Design review of the part built by this model. Coordinates are the model's own, in mm. A direction names the side the tool comes from. Coordinates: 2 decimals unless noted, no trailing zeros. Loops run counter-clockwise (first coordinate to the right, second up) from the corner with the lowest first, then second, coordinate; pieces in that order, holes last.
Q1. Add section C-C on x = 31.5. Give the boundary of the cut face in (y, z).
Q2. Draft analysis for pull direction X (two halves, no side actions). For faces 3 (the face through (2.85, 3.19, -81.99)), 4 (the face through (42.3, 0.4, -5)), 5 (the face through (7.008, 3.901, -40.115)), state which applies: released by +X, released by -X, zero draft, split by the parting line, or undercut.
Q3. For P1, Ø1.5, axis at x = 75, y = 4.5, coming from the +Z side; P2, Ø2, axis at x = 76.5, y = 2, coming from the +Z side, all flat-tipped, find the tip position at first contact; note any pin that passes through.
Q4. Add section D-D on y = 3.15. Give the boundary of the cut face in (x, z).
Q5. Add section B-B on z = -16.5. Give the boundary of the cut face in (x, y), and give its area (3 significant figures).
Q6. Wall thickness on probe 1 along X at (y, z) = (4.5, -50); probe 2 along Y at (x, z) = (4, -42.5); probe 3 along X at (y, z) = (4.5, -11.5): over which ranges is each line inside the solid? List them lowest first.
Q7. Machinability: for faces 1 (the face through (85, 3, -47)), 2 (the face through (22.92, 3.19, -23.91)), which of the approach directions +Z, -Z, +X, -X, +Y, -Y give a long, thin tool a straight path to every point of the face, cutting with its end or side? Answer none if there is none.
Q8. Add section A-A on x = 42.5. Give the boundary of the cut face in (y, z).
```python
from build123d import *

# Parameters (mm, degrees)
SKETCH1_W           = 85
SKETCH1_H           = 85
BOSS_EXTRUDE1_DEPTH = 6.3
CUT_EXTRUDE1_DEPTH  = 10
SKETCH3_R           = 2.5
CUT_EXTRUDE2_DEPTH  = 86
SKETCH4_R           = 2.5
CUT_EXTRUDE3_DEPTH  = 86
FILLET1_R           = 20
FILLET2_R           = 10


with BuildPart() as part:
    # Sketch1 → Boss-Extrude1 (new body)
    with BuildSketch(Plane(origin=(0, 0, 0), x_dir=(1, 0, 0), z_dir=(0, 1, 0))):
        with Locations((42.5, 42.5)):
            Rectangle(SKETCH1_W, SKETCH1_H)
    extrude(amount=BOSS_EXTRUDE1_DEPTH)

    # Sketch2 → Cut-Extrude1 (cut)
    with BuildSketch(Plane(origin=(0, 6.3, 0), x_dir=(1, 0, 0), z_dir=(0, 1, 0))):
        with BuildLine():
            Line((16.519237886, 35), (29.509618943, 12.5))
            ThreePointArc((29.509618943, 12.5), (42.5, 5), (55.490381057, 12.5))
            Line((55.490381057, 12.5), (68.480762114, 35))
            ThreePointArc((68.480762114, 35), (42.5, 80), (16.519237886, 35))
        make_face()
    extrude(amount=-CUT_EXTRUDE1_DEPTH, mode=Mode.SUBTRACT)

    # Sketch3 → Cut-Extrude2 (cut, through all)
    with BuildSketch(Plane.XY):
        with Locations((42.5, 3.15)):
            Circle(SKETCH3_R)
    extrude(amount=-CUT_EXTRUDE2_DEPTH, mode=Mode.SUBTRACT)

    # Sketch4 → Cut-Extrude3 (cut, through all)
    with BuildSketch(Plane.ZY):
        with Locations((-42.5, 3.15)):
            Circle(SKETCH4_R)
    extrude(amount=-CUT_EXTRUDE3_DEPTH, mode=Mode.SUBTRACT)

    # Fillet1
    fillet1_edges = [part.edges().sort_by_distance(p)[0] for p in [
        (85, 3.15, 0),
        (0, 3.15, 0),
    ]]
    fillet(fillet1_edges, radius=FILLET1_R)

    # Fillet2
    fillet2_edges = [part.edges().sort_by_distance(p)[0] for p in [
        (0, 3.15, -85),
        (85, 3.15, -85),
    ]]
    fillet(fillet2_edges, radius=FILLET2_R)


solid = part.part
```
Entries:
1. outline: (0, -85) - (6.3, -85) - (6.3, -77.91) - (0, -77.91) - close; (0, -9.8) - (6.3, -9.8) - (6.3, 0) - (0, 0) - close
2. face 3: released by -X
2. face 4: undercut
2. face 5: zero draft
3. P1: stops at z = -2.27
3. P2: stops at z = -2.98
4. outline: (0, -75) arc R10 ccw to (10, -85) - (40, -85) - (40, -79.9) arc R30 cw to (12.92, -45) - (0, -45) - close; (0, -40) - (14.22, -40) arc R30 cw to (16.52, -35) - (29.51, -12.5) arc R15 cw to (40, -5.21) - (40, 0) - (20, 0) arc R20 ccw to (0, -20) - close; (45, -85) - (75, -85) arc R10 ccw to (85, -75) - (85, -45) - (72.08, -45) arc R30 cw to (45, -79.9) - close; (45, -5.21) arc R15 cw to (55.49, -12.5) - (68.48, -35) arc R30 cw to (70.78, -40) - (85, -40) - (85, -20) arc R20 ccw to (65, 0) - (45, 0) - close
5. outline: (0.31, 0) - (27.2, 0) - (27.2, 6.3) - (0.31, 6.3) - close; (57.8, 0) - (84.69, 0) - (84.69, 6.3) - (57.8, 6.3) - close
5. area: 339 mm2
6. probe 1: x = 0 to 12.5, 72.5 to 85
6. probe 2: y = 0 to 0.65, 5.65 to 6.3
6. probe 3: x = 1.9 to 30.14, 54.86 to 83.1
7. face 1: +Z, -Z, +X, +Y, -Y
7. face 2: +Y, -Y
8. outline: (0, -85) - (0.65, -85) - (0.65, -80) - (0, -80) - close; (0, -5) - (0.65, -5) - (0.65, 0) - (0, 0) - close; (5.65, -85) - (6.3, -85) - (6.3, -80) - (5.65, -80) - close; (5.65, -5) - (6.3, -5) - (6.3, 0) - (5.65, 0) - close
